```python
from build123d import *

# Parameters (mm, degrees)
F0_R     = 3
F1_DEPTH = 18
F2_DEPTH = 14
F3_DEPTH = 12.5


# Not quite as in the source:
# - ends of sketch curves that miss each other by under 0.0002 mm in the source are joined


with BuildPart() as f1:
    # F0 (on Front) → F1 (new body)
    with BuildSketch(Plane.XZ):
        with BuildLine():
            Line((-119.3285324557, -448.2617723394), (-101.6685144557, -441.5452453394))
            ThreePointArc((-101.6685144557, -441.5452453394), (-97.1422559669, -438.0887567531), (-95.2370421293, -432.7217753041))
            Line((-95.2370421293, -432.7217753041), (-58.8235234557, 262.0895416606))
            ThreePointArc((-58.8235234557, 262.0895416606), (-58.06143799, 264.2363343101), (-56.250934498, 265.6189297718))
            Line((-56.250934498, 265.6189297718), (85.2578445443, 319.4380986606))
            Line((85.2578445443, 319.4380986606), (41.3370915443, 363.9049416606))
            Line((41.3370915443, 363.9049416606), (-132.8833544557, 297.6447436606))
            Line((-132.8833544557, 297.6447436606), (-132.8833544557, -438.9149423394))
            ThreePointArc((-132.8833544557, -438.9149423394), (-128.5601395631, -447.1474456551), (-119.3285324557, -448.2617723394))
        make_face()
        with Locations((-116.1363294557, -390.4994083394)):
            Circle(F0_R, mode=Mode.SUBTRACT)
        with Locations((-113.3511164557, -246.7075803394)):
            Circle(F0_R, mode=Mode.SUBTRACT)
        with Locations((-107.9187374557, -78.3756793394)):
            Circle(F0_R, mode=Mode.SUBTRACT)
        with Locations((-105.9467734557, 128.6347116606)):
            Circle(F0_R, mode=Mode.SUBTRACT)
        with Locations((-99.7011464557, 233.7480486606)):
            Circle(F0_R, mode=Mode.SUBTRACT)
        with Locations((-120.2235504557, 275.4892296606)):
            Circle(F0_R, mode=Mode.SUBTRACT)
        with BuildLine():
            ThreePointArc((-90.3754553764, 255.7239337355), (-90.5472879726, 250.0640248228), (-96.2068413545, 250.2471937553))
            Line((-96.2068413545, 250.2471937553), (-102.4861304557, 250.4567146606))
            ThreePointArc((-102.4861304557, 250.4567146606), (-108.1617141765, 250.6689360163), (-107.9038666822, 256.3426299107))
            Line((-107.9038666822, 256.3426299107), (-107.0299454557, 291.0352376606))
            ThreePointArc((-107.0299454557, 291.0352376606), (-106.7545815371, 296.6558621202), (-101.1313975225, 296.4389595982))
            Line((-101.1313975225, 296.4389595982), (-94.4508164557, 296.2088706606))
            ThreePointArc((-94.4508164557, 296.2088706606), (-88.7851572097, 296.0073908544), (-89.0114747479, 290.3426689785))
            Line((-89.0114747479, 290.3426689785), (-90.3754553764, 255.7239337355))
        make_face(mode=Mode.SUBTRACT)
        with Locations((-42.3545774557, 288.6199666606)):
            Circle(F0_R, mode=Mode.SUBTRACT)
        with Locations((51.7271015443, 324.4037386606)):
            Circle(F0_R, mode=Mode.SUBTRACT)
        with Locations((-116.1363294557, -390.4994083394)):
            Circle(F0_R)
        with Locations((-113.3511164557, -246.7075803394)):
            Circle(F0_R)
        with Locations((-107.9187374557, -78.3756793394)):
            Circle(F0_R)
        with Locations((-105.9467734557, 128.6347116606)):
            Circle(F0_R)
        with Locations((-120.2235504557, 275.4892296606)):
            Circle(F0_R)
        with Locations((-99.7011464557, 233.7480486606)):
            Circle(F0_R)
        with Locations((-42.3545774557, 288.6199666606)):
            Circle(F0_R)
        with Locations((51.7271015443, 324.4037386606)):
            Circle(F0_R)
        with BuildLine():
            Line((-102.4861304557, 250.4567146606), (-96.2068414557, 250.2471936606))
            ThreePointArc((-96.2068414557, 250.2471936606), (-90.5472879726, 250.0640248228), (-90.3754553764, 255.7239337355))
            Line((-90.3754553764, 255.7239337355), (-89.0114744557, 290.3426686606))
            ThreePointArc((-89.0114744557, 290.3426686606), (-88.7851572097, 296.0073908544), (-94.4508168599, 296.2088710928))
            Line((-94.4508168599, 296.2088710928), (-101.1313974557, 296.4389596606))
            ThreePointArc((-101.1313974557, 296.4389596606), (-106.7545815371, 296.6558621202), (-107.0299455087, 291.0352376131))
            Line((-107.0299455087, 291.0352376131), (-107.9038664557, 256.3426296606))
            ThreePointArc((-107.9038664557, 256.3426296606), (-108.1617141765, 250.6689360163), (-102.4861304557, 250.4567146606))
        make_face()
    extrude(amount=-F1_DEPTH)

    # F0 (on Front) → F2 (cut)
    with BuildSketch(Plane.XZ):
        with Locations((-116.1363294557, -390.4994083394)):
            Circle(F0_R)
        with Locations((-113.3511164557, -246.7075803394)):
            Circle(F0_R)
        with Locations((-107.9187374557, -78.3756793394)):
            Circle(F0_R)
        with Locations((-105.9467734557, 128.6347116606)):
            Circle(F0_R)
        with Locations((-120.2235504557, 275.4892296606)):
            Circle(F0_R)
        with Locations((-99.7011464557, 233.7480486606)):
            Circle(F0_R)
        with Locations((-42.3545774557, 288.6199666606)):
            Circle(F0_R)
        with Locations((51.7271015443, 324.4037386606)):
            Circle(F0_R)
    extrude(amount=-F2_DEPTH, mode=Mode.SUBTRACT)

    # F0 (on Front) → F3 (cut)
    with BuildSketch(Plane.XZ):
        with BuildLine():
            Line((-102.4861304557, 250.4567146606), (-96.2068414557, 250.2471936606))
            ThreePointArc((-96.2068414557, 250.2471936606), (-90.5472879726, 250.0640248228), (-90.3754553764, 255.7239337355))
            Line((-90.3754553764, 255.7239337355), (-89.0114744557, 290.3426686606))
            ThreePointArc((-89.0114744557, 290.3426686606), (-88.7851572097, 296.0073908544), (-94.4508168599, 296.2088710928))
            Line((-94.4508168599, 296.2088710928), (-101.1313974557, 296.4389596606))
            ThreePointArc((-101.1313974557, 296.4389596606), (-106.7545815371, 296.6558621202), (-107.0299455087, 291.0352376131))
            Line((-107.0299455087, 291.0352376131), (-107.9038664557, 256.3426296606))
            ThreePointArc((-107.9038664557, 256.3426296606), (-108.1617141765, 250.6689360163), (-102.4861304557, 250.4567146606))
        make_face()
    extrude(amount=-F3_DEPTH, mode=Mode.SUBTRACT)


solid = f1.part
```
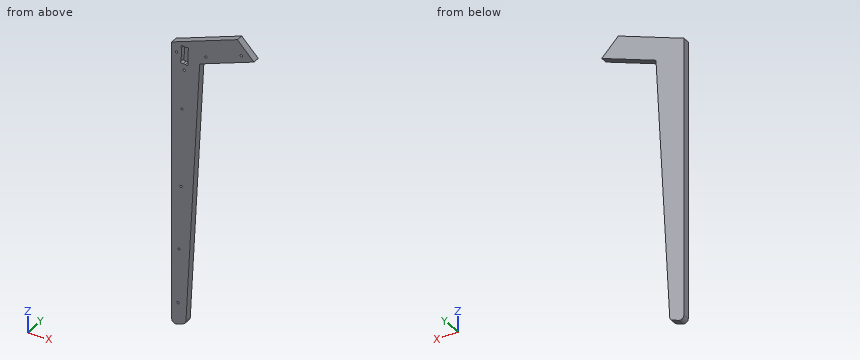
Build history of the part. All positions in model axes, mm. Give positions to 0.01 mm unless a question says otherwise; leave off trailing zeros. Loops run counter-clockwise (first coordinate to the right, second up) from the corner with the lowest first, then second, coordinate; pieces in that order, holes last.
1) Band-saw the part on C-C on x = -5.5. List the corners of the cut face in (y, z), then the cut area to 3 significant figures.
Values follow:
outline: (0, 284.92) - (18, 284.92) - (18, 346.09) - (0, 346.09) - close
area: 1,100 mm2
2) Band-saw the part on A-A on y = 5.25. State how many separate pieces and enclosed holes the cut face has, then the cut area to 3 significant figures.
Values follow:
separate pieces: 1
enclosed holes: 9
area: 49,300 mm2
3) Drop flat-ended pins along their axis: P1, Ø5.5, axis at x = -99.7, z = 233.75, coming from the -Y side; P2, Ø11, axis at x = -101.5, z = 275, coming from the -Y side. Give the stop position or say it passes through.
Values follow:
P1: stops at y = 14
P2: stops at y = 12.5
4) Band-saw the part on B-B on z = -107.5. List the corners of the cut face in (x, y).
Values follow:
outline: (-132.88, 0) - (-78.19, 0) - (-78.19, 18) - (-132.88, 18) - close
5) Probe line 1 along X through (y, z) = (3, -290); line 2 along X through (y, z) = (5.5, -53); line 3 along Z through (x, y) = (-21, 12.25). List the from-to ranges inside material, lowest first.
Values follow:
line 1: x = -132.88 to -87.76
line 2: x = -132.88 to -75.34
line 3: z = 279.03 to 340.2
